The model under review builds one solid part; all positions refer to its coordinate system, in mm. A direction names the side the tool comes from. Coordinates: 2 decimals unless noted, no trailing zeros. Loops run counter-clockwise (first coordinate to the right, second up) from the corner with the lowest first, then second, coordinate; pieces in that order, holes last. Notation, with made-up numbers: M 83.5,55.25 L 142.5,55.25 A21 ccw 142.5,61.25 Z; hole C 28.25,62 d9. An arc over 180 degrees is marked long. Use one line per item in the form item = value.
Autodesk Inventor part; units mm, degrees
ref_plane "YZ Plane" through (0, 0, 0) normal (1, 0, 0) x (0, 1, 0)
ref_plane "XZ Plane" through (0, 0, 0) normal (0, 1, 0) x (-1, 0, 0)
ref_plane "XY Plane" through (0, 0, 0) normal (0, 0, 1) x (1, 0, 0)
sketch "Sketch1" plane through (0, 0, 0) normal (0, 1, 0) x (-1, 0, 0)
  line L0 (0, 0) -> (53.34, 0)
  line L1 (53.34, 0) -> (53.34, -60.2234)
  line L2 (53.34, -60.2234) -> (0, -60.2234)
  line L3 (0, -60.2234) -> (0, 0)
  dimension "d0" = 53.34
  dimension "d1" = 60.2234
extrude "Extrusion1" add sketch "Sketch1" along normal blind 1.397
fillet "Fillet1" radius 3.175 4 edges at (0, 0.6985, -60.2234) (-53.34, 0.6985, -60.2234) (0, 0.6985, 0) (-53.34, 0.6985, 0)
sketch "Sketch2" plane through (0, 1.397, 0) normal (0, 1, 0) x (1, 0, 0)
  line L0 (0, 0) -> (-74.2846, 0) construction
  line L1 (0, 0) -> (0, 92.3898) construction
  line L2 (-3.9116, 10.795) -> (-1.3716, 10.795)
  line L3 (-1.3716, 10.795) -> (-1.3716, 49.2506)
  line L4 (-1.3716, 49.2506) -> (-3.9116, 49.2506)
  line L5 (-3.9116, 49.2506) -> (-3.9116, 10.795)
  line L6 (-51.9684, 1.778) -> (-49.4284, 1.778)
  line L7 (-49.4284, 1.778) -> (-49.4284, 48.8569)
  line L8 (-49.4284, 48.8569) -> (-51.9684, 48.8569)
  line L9 (-51.9684, 48.8569) -> (-51.9684, 1.778)
  line L10 (-53.34, 57.0484) -> (-53.34, 3.175)
  line L11 (-53.34, 50.5823) -> (-53.34, -10.1143) construction
  dimension "d5" = 2.54
  dimension "d6" = 2.54
  dimension "d7" = 38.4556
  dimension "d8" = 47.0789
  dimension "d9" = 1.778
  dimension "d10" = 3.9116
  dimension "d11" = 10.795
  dimension "d12" = 3.9116
extrude "Extrusion2" add sketch "Sketch2" along normal blind 8.636
sketch "Sketch3" plane through (0, 1.397, 0) normal (0, 1, 0) x (1, 0, 0)
  line L0 (0, 0) -> (-18.0314, 0) construction
  line L1 (-50.165, 0) -> (-3.175, 0)
  line L2 (0, 0) -> (0, 13.9144) construction
  line L3 (0, 3.175) -> (0, 57.0484)
  line L4 (-15.3162, -3.556) -> (-6.477, -3.556)
  line L5 (-6.477, -3.556) -> (-6.477, 10.668)
  line L6 (-6.477, 10.668) -> (-15.3162, 10.668)
  line L7 (-15.3162, 10.668) -> (-15.3162, -3.556)
  dimension "d19" = 8.8392
  dimension "d20" = 14.224
  dimension "d21" = 3.556
  dimension "d22" = 6.477
extrude "Extrusion3" add sketch "Sketch3" along normal blind 10.8839
sketch "Sketch4" plane through (0, 0, 0) normal (0, -1, 0) x (1, 0, 0)
  line L0 (0, 0) -> (0, -16.5285) construction
  line L1 (0, -3.175) -> (0, -57.0484)
  line L2 (0, 0) -> (-10.3791, 0) construction
  line L3 (-3.175, 0) -> (-50.165, 0)
  line L4 (-49.4284, -48.8569) -> (-49.4284, -1.778)
  line L5 (-51.9684, -1.778) -> (-51.9684, -48.8569)
  line L6 (-49.4284, -1.778) -> (-51.9684, -1.778)
  line L7 (-51.9684, -1.778) -> (-51.9684, -48.8569)
  line L8 (-51.9684, -48.8569) -> (-49.4284, -48.8569)
  line L9 (-49.4284, -48.8569) -> (-49.4284, -1.778)
  line L10 (-1.3716, -10.795) -> (-3.9116, -10.795)
  line L11 (-3.9116, -10.795) -> (-3.9116, -49.2506)
  line L12 (-3.9116, -49.2506) -> (-1.3716, -49.2506)
  line L13 (-1.3716, -49.2506) -> (-1.3716, -10.795)
  dimension "d25" = 47.0789
  dimension "d27" = 2.54
  dimension "d28" = 38.4556
  dimension "d29" = 10.795
  dimension "d30" = 3.9116
  dimension "d31" = 1.778
extrude "Extrusion4" add sketch "Sketch4" along normal blind 13.1572
sketch "Sketch5" plane through (-15.3162, 1.397, 3.556) normal (0, 0, 1) x (1, 0, 0)
  circle A0 centre (4.4196, 6.4389) radius 3.175
  line L0 (0, 10.8839) -> (8.8392, 10.8839)
  line L1 (4.4196, 10.8839) -> (4.4196, -0.1131) construction
  point P0 (15.3162, -1.397)
  dimension "d34" = 6.35
  dimension "d35" = 4.445
extrude "Extrusion5" cut sketch "Sketch5" against normal blind 6.35
properties part number "board_mockup"
1. The part is to be moulded in two halves that separate along X. For faces 4 (the face through (-3, 6, -10.795)), 5 (the face through (-1.372, 6, -30)), 6 (the face through (-26, 1.397, -30)), 7 (the face through (-51.968, -6, -25)), say which applies: pulls with the +X half, pulls with the -X half, needs draft (parallel to the pull), parting line crosses it, or undercut.
Response values:
face_4 = needs draft
face_5 = pulls with the +X half
face_6 = undercut
face_7 = pulls with the -X half
2. Insertion check: P1, Ø5.5, axis at y = 9, z = -1.5, coming from the -X side; P2, Ø14.5, axis at y = -9, z = -24, coming from the +X side; P3, Ø3, axis at x = -50.5, y = -4.5, coming from the -Z side; P4, Ø1, axis at y = 1, z = -30, coming from the +X side. Each pin has a flat end and moves straight along its axis. Give the tip position at first contact, or say it passes through.
Response values:
P1 = -51.97
P2 = -1.37
P3 = -48.86
P4 = 0
3. Add section C-C (x = -5.5). State the section outline as (y, z) points, then the cut area to 3 significant figures.
Response values:
outline = M 0,-60.22 L 1.4,-60.22 L 1.4,0 L 0,0 Z
area = 84.1 mm^2
4. Add section A-A (y = -7.5). State the section outline as (x, z) points (3 decimals).
Response values:
outline = M -51.968,-48.857 L -49.428,-48.857 L -49.428,-1.778 L -51.968,-1.778 Z; M -3.912,-49.251 L -1.372,-49.251 L -1.372,-10.795 L -3.912,-10.795 Z
5. Add section D-D (y = 8.75). State the section outline as (x, z) points (3 decimals), then the cut area to 3 significant figures.
Response values:
outline = M -51.968,-48.857 L -49.428,-48.857 L -49.428,-1.778 L -51.968,-1.778 Z; M -15.316,-10.668 L -6.477,-10.668 L -6.477,3.556 L -7.856,3.556 L -7.856,-2.794 L -13.937,-2.794 L -13.937,3.556 L -15.316,3.556 Z; M -3.912,-49.251 L -1.372,-49.251 L -1.372,-10.795 L -3.912,-10.795 Z
area = 304 mm^2
6. Wall thickness on line 1 along X through (y, z) = (-11.75, -29.5); line 2 along Y through (x, z) = (-27, -34.5); line 3 along Z through (x, y) = (-49.5, 10): over which ranges is each line inside the solid? List them lowest first. Write a range as from..to.
Response values:
line_1 = -51.97..-49.43, -3.91..-1.37
line_2 = 0..1.4
line_3 = -48.86..-1.78
7. Machinability: for faces 1 (the face through (-1.372, -6, -30)), 2 (the face through (-51, 6, -1.778)), 3 (the face through (-11, 1.397, 2)), which of the approach directions +Z, -Z, +X, -X, +Y, -Y give a long, thin tool a straight path to every point of the face, cutting with its end or side? Answer none if there is none.
Response values:
face_1 = +Z, -Z, +X, -Y
face_2 = +Z, -X, +Y
face_3 = +Z, +X, -X, -Y
8. Add section B-B (z = -22). State the section outline as (x, y) points.
Response values:
outline = M -53.34,0 L -51.97,0 L -51.97,-13.16 L -49.43,-13.16 L -49.43,0 L -3.91,0 L -3.91,-13.16 L -1.37,-13.16 L -1.37,0 L 0,0 L 0,1.4 L -1.37,1.4 L -1.37,10.03 L -3.91,10.03 L -3.91,1.4 L -49.43,1.4 L -49.43,10.03 L -51.97,10.03 L -51.97,1.4 L -53.34,1.4 Z
